from build123d import *

# Parameters (mm, degrees)
FILLET1_R             = 0.2
RECPAT_COUNT          = 2
RECPAT_ANGLE          = 90
CHAMFER_1_SIZE        = 0.5
CUT_EXTRUDE_START     = -1.932317225
CUT_EXTRUDE_1_DEPTH   = 0.992538955
CUT_EXTRUDE_1_2_DEPTH = 0.992538955
CUT_EXTRUDE_1_3_DEPTH = 0.992538955
CUT_EXTRUDE_1_4_DEPTH = 0.992538955


# Read off the part's stored shape, not the designer's step: Вытянуть1
with BuildPart() as part:
    # BodySke → Base-Revolve (revolve)
    with BuildSketch(Plane.XY, mode=Mode.PRIVATE) as base_revolve_sk:
        Polygon((3.05, 2), (3.05, 5), (2.05, 5), (2.05, 0), (19.05, 0), (19.05, 2), align=None)
    revolve(base_revolve_sk.sketch.rotate(Axis((-6.35, 0, 0), (1, 0, 0)), 90), axis=Axis((-6.35, 0, 0), (1, 0, 0)))

    # Fillet1
    fillet1_edges = [part.edges().sort_by_distance(p)[0] for p in [
        (3.05, 0, -2),
    ]]
    fillet(fillet1_edges, radius=FILLET1_R)

    # PanSke → Pan (revolve)
    with BuildSketch(Plane.XY):
        with BuildLine():
            Line((2.05, 4.424646879), (2.05, 0))
            Line((2.05, 0), (0, 0))
            ThreePointArc((0, 0), (0.537396082, 2.438237068), (2.05, 4.424646879))
        make_face()
    revolve(axis=Axis((0, 0, 0), (1, 0, 0)))

    # Sketch3 → Recess section 0
    with BuildSketch(Plane(origin=(0, 0, 0), x_dir=(0, 0, -1), z_dir=(1, 0, 0))):
        with BuildLine():
            Line((-0.515, 2.15), (0.515, 2.15))
            Line((0.515, 2.15), (0.515, -2.15))
            Line((0.515, -2.15), (-0.515, -2.15))
            Line((-0.515, -2.15), (-0.515, 2.15))
        make_face()
    # Sketch4 → Recess section 1
    with BuildSketch(Plane(origin=(2.34, 0, 0), x_dir=(0, 0, -1), z_dir=(1, 0, 0))):
        with BuildLine():
            Line((-0.37, 1.45), (0.37, 1.45))
            Line((0.37, 1.45), (0.37, -1.45))
            Line((0.37, -1.45), (-0.37, -1.45))
            Line((-0.37, -1.45), (-0.37, 1.45))
        make_face()
    recess = loft(mode=Mode.SUBTRACT)

    # RecPat: Recess ×2 about axis
    recpat_axis = Axis((0, 0, 0), (1, 0, 0))
    for i in range(1, RECPAT_COUNT):
        add(recess.rotate(recpat_axis, i * RECPAT_ANGLE / (RECPAT_COUNT - 1)), mode=Mode.SUBTRACT)

    # RecCorSke → RecessCore (revolve, cut)
    with BuildSketch(Plane.XY, mode=Mode.PRIVATE) as recesscore_sk:
        Polygon((0, 0), (0, 1.032809711), (2.6, 0.851), (2.876506661, 0), align=None)
    revolve(recesscore_sk.sketch.rotate(Axis((-3.175, 0, 0), (1, 0, 0)), 90), axis=Axis((-3.175, 0, 0), (1, 0, 0)), mode=Mode.SUBTRACT)

    # Фаска1
    chamfer_1_edges = [part.edges().sort_by_distance(p)[0] for p in [
        (19.05, 0, -2),
    ]]
    chamfer(chamfer_1_edges, length=CHAMFER_1_SIZE)

    # Вытянуть1 outline → Вытянуть1 (cut)
    with BuildSketch(Plane(origin=(0, 0, 0), x_dir=(0.9932989193126689, -0.08172287590474257, -0.08172287590474261), z_dir=(0.1155735994606204, 0.7023684015912574, 0.7023684015912578)).offset(CUT_EXTRUDE_START)):
        Polygon((-1, -0.919204654), (0.206895578, -0.216114133), (0.577867997, 0), (0.206895578, 0.216114133), (-1, 0.919204654), align=None)
    extrude(amount=CUT_EXTRUDE_1_DEPTH, mode=Mode.SUBTRACT)

    # Cut-Extrude 1 2 outline → Cut-Extrude 1 2 (cut)
    with BuildSketch(Plane(origin=(0, 0, 0), x_dir=(0.9932989193126689, -0.08172287590474257, 0.08172287590474261), z_dir=(0.1155735994606204, 0.7023684015912574, -0.7023684015912578)).offset(CUT_EXTRUDE_START)):
        Polygon((0.206895578, -0.216114133), (0.577867997, 0), (0.206895578, 0.216114133), (-1, 0.919204654), (-1, -0.919204654), align=None)
    extrude(amount=CUT_EXTRUDE_1_2_DEPTH, mode=Mode.SUBTRACT)

    # Cut-Extrude 1 3 outline → Cut-Extrude 1 3 (cut)
    with BuildSketch(Plane(origin=(0, 0, 0), x_dir=(0.9932989193126689, 0.08172287590474257, 0.08172287590474261), z_dir=(0.1155735994606204, -0.7023684015912574, -0.7023684015912578)).offset(CUT_EXTRUDE_START)):
        Polygon((0.206895578, -0.216114133), (0.577867997, 0), (0.206895578, 0.216114133), (-1, 0.919204654), (-1, -0.919204654), align=None)
    extrude(amount=CUT_EXTRUDE_1_3_DEPTH, mode=Mode.SUBTRACT)

    # Cut-Extrude 1 4 outline → Cut-Extrude 1 4 (cut)
    with BuildSketch(Plane(origin=(0, 0, 0), x_dir=(0.9932989193126689, 0.08172287590474257, -0.08172287590474261), z_dir=(0.1155735994606204, -0.7023684015912574, 0.7023684015912578)).offset(CUT_EXTRUDE_START)):
        Polygon((-1, -0.919204654), (0.206895578, -0.216114133), (0.577867997, 0), (0.206895578, 0.216114133), (-1, 0.919204654), align=None)
    extrude(amount=CUT_EXTRUDE_1_4_DEPTH, mode=Mode.SUBTRACT)


solid = part.part
CAD build for the part. Positions are in the model's coordinates, mm. Round coordinates to 2 decimals unless told otherwise and drop trailing zeros. Order: outer loops, then holes, each group sorted by start corner. A loop starts at its lowest first (then second) coordinate and runs counter-clockwise, first axis right, second up. Notation, with made-up numbers: M 24.25,53 L 39.25,53 A12 cw 39.25,76 Z; hole C 81.5,60.5 d1. An arc over 180 degrees is marked long. Use one line per item in the form item = value.
Q1. Flat gauge pins, fed straight in: P1, Ø6, axis at x = 7, z = 2.5, coming from the +Y side; P2, Ø1, axis at y = 2, z = 2, coming from the +X side; P3, Ø2, axis at x = 13, y = 0, coming from the +Z side. Where does each tip first touch, or does it go through?
Recorded:
P1 = 2
P2 = 3.05
P3 = 2
Q2. Two-plate mould, pull along Y, no slides. Class faces 1 (the flat face through (3.05, 1, -2.2)), 2 (the cylindrical face through (11, 2, 0)), 3 (the conical face through (1.6, -0.6, -0.7)), 4 (the conical face through (2.863, -0.012, 0.039)): +Y half, -Y half, draft (parallel to the pull), parting line (faces both ways), or undercut.
Recorded:
face_1 = draft
face_2 = parting line
face_3 = undercut
face_4 = undercut
Q3. Saw through at C-C on z = 3. Give the cut face in (x, y), then the cut area to 3 significant figures.
Recorded:
outline = M 2.05,-4 L 3.05,-4 L 3.05,4 L 2.05,4 L 2.05,3.25 A4.96 ccw 2.05,-3.25 Z
area = 13.4 mm^2
Q4. Saw through at B-B on y = -3.25. Give the cut face in (x, z), then the cut area to 3 significant figures.
Recorded:
outline = M 2.05,-3.8 L 3.05,-3.8 L 3.05,3.8 L 2.05,3.8 L 2.05,3 A4.8 ccw 2.05,-3 Z
area = 11.9 mm^2
Q5. Probe L1, parallel to X at y = 0.75, z = 3; L2, parallel to X at y = -2.75, z = -3.75; L3, parallel to Z at x = 1, y = 0.25. List the from-to ranges inside material, lowest first.
Recorded:
L1 = 0.89 to 3.05
L2 = 2.05 to 3.05
L3 = -3.25 to -1.85, 1.85 to 3.25
Q6. Saw through at A-A on x = 13.5. Give the cut face in (y, z).
Recorded:
outline = C 0,0 d4
